Input: part model. Units: mm. Frame: model coordinates. A direction names the side the tool comes from. Coordinates: 2 decimals unless noted, no trailing zeros. Order: outer loops, then holes, each group sorted by start corner. A loop starts at its lowest first (then second) coordinate and runs counter-clockwise, first axis right, second up. Notation, with made-up numbers: (88, -22.5) - (101, -22.5) arc R16 cw to (101, -13.5) - close; hole circle Ø2 at (-16, 75.5). An arc over 180 degrees is marked (long way). Use a Markdown table: item, result. Add a question column.
Autodesk Inventor part; units mm, degrees
ref_plane "Work Plane1" through (0, 0, 46) normal (1, 0, 0) x (0, 0, -1)
ref_plane "YZ Plane" through (0, 0, 0) normal (1, 0, 0) x (0, 1, 0)
ref_plane "XZ Plane" through (0, 0, 0) normal (0, 1, 0) x (-1, 0, 0)
sketch "Sketch1" plane through (0, 0, 0) normal (0, 1, 0) x (-1, 0, 0)
  line L0 (-66, 49) -> (66, 49)
  line L1 (69, 46) -> (69, -46)
  line L2 (66, -49) -> (-66, -49)
  line L3 (-69, -46) -> (-69, 46)
  line L4 (-69, 49) -> (69, -49) construction
  line L5 (69, 49) -> (-69, -49) construction
  arc A0 (69, 46) -> (66, 49) centre (66, 46) ccw
  arc A1 (-66, 49) -> (-69, 46) centre (-66, 46) ccw
  arc A2 (-69, -46) -> (-66, -49) centre (-66, -46) ccw
  arc A3 (66, -49) -> (69, -46) centre (66, -46) ccw
  line L6 (65.5, -42.5) -> (65.5, 42.5)
  line L7 (62.5, 45.5) -> (-62.5, 45.5)
  line L8 (-65.5, 42.5) -> (-65.5, -42.5)
  line L9 (-62.5, -45.5) -> (62.5, -45.5)
  arc A4 (65.5, 42.5) -> (62.5, 45.5) centre (62.5, 42.5) ccw
  arc A5 (-62.5, 45.5) -> (-65.5, 42.5) centre (-62.5, 42.5) ccw
  arc A6 (-65.5, -42.5) -> (-62.5, -45.5) centre (-62.5, -42.5) ccw
  arc A7 (62.5, -45.5) -> (65.5, -42.5) centre (62.5, -42.5) ccw
  point P0 (0, 0)
  dimension "d0" = 138
  dimension "d1" = 98
  dimension "d2" = 3
  dimension "d3" = 3.5
  dimension "d4" = 3
extrude "Extrusion1" add sketch "Sketch1" along normal blind 3.5 contours A7 L9 A6 L8 A5 L7 A4 L6
extrude "Extrusion2" add sketch "Sketch1" along normal blind 42
sketch "Sketch2" plane through (0, 3.5, 0) normal (0, 1, 0) x (1, 0, 0)
  circle A0 centre (-14.4905, 21.8769) radius 1.5
  line L0 (-17.4775, 25.0064) -> (63, 25.0064)
  line L1 (-17.4775, -25.0064) -> (-17.4775, 25.0064)
  circle A1 centre (-14.4905, -22.0231) radius 1.5
  line L2 (63, -25.0064) -> (-17.4775, -25.0064)
  circle A2 centre (60.3095, -22.0231) radius 1.5
  line L3 (63, 25.0064) -> (63, -25.0064)
  circle A3 centre (60.3095, 21.8769) radius 1.5
  line L4 (-62.5, -45.5) -> (62.5, -45.5)
  circle A4 centre (-14.4905, -22.0231) radius 4.5
  circle A5 centre (-14.4905, 21.8769) radius 4.5
  circle A6 centre (60.3095, 21.8769) radius 4.5
  circle A7 centre (60.3095, -22.0231) radius 4.5
  arc A8 (-65.5, -42.5) -> (-62.5, -45.5) centre (-62.5, -42.5) ccw
  line L5 (-62.5, -45.5) -> (62.5, -45.5)
  arc A9 (62.5, -45.5) -> (65.5, -42.5) centre (62.5, -42.5) ccw
  line L6 (65.5, -42.5) -> (65.5, 42.5)
  arc A10 (65.5, 42.5) -> (62.5, 45.5) centre (62.5, 42.5) ccw
  line L7 (62.5, 45.5) -> (-62.5, 45.5)
  arc A11 (-62.5, 45.5) -> (-65.5, 42.5) centre (-62.5, 42.5) ccw
  line L8 (-65.5, 42.5) -> (-65.5, -42.5)
  line L9 (-65.5, -42.5) -> (-65.5, 42.5)
  line L10 (-65.5, 0) -> (-27.8028, 0)
  point P0 (0, 0)
  point P1 (22.7612, -25.0064)
  point P2 (-17.4775, 0)
  dimension "d9" = 3
  dimension "d10" = 80.4775
  dimension "d11" = 50.0127
  dimension "d14" = 2.6905
  dimension "d15" = 46.8833
  dimension "d16" = 2.6905
  dimension "d17" = 2.9833
  dimension "d18" = 77.4905
  dimension "d19" = 46.8833
  dimension "d20" = 77.4905
  dimension "d21" = 2.9833
  dimension "d23" = 9
  dimension "d24" = 9
  dimension "d25" = 9
  dimension "d26" = 9
  dimension "d59" = 2.5
extrude "Extrusion3" add sketch "Sketch2" along normal blind 15 contours L1 A5 L0 | L0 A5 L1 | A6 L3 L0 | L0 L3 A6 | A4 L2 L1 | L1 L2 A4 | A7 L2 L3 | L3 L2 A7
sketch "Sketch4" plane through (0, 3.5, 0) normal (0, 1, 0) x (1, 0, 0)
  circle A0 centre (-43.1118, 27.6225) radius 1.5
  circle A1 centre (-43.1118, -27.6225) radius 1.5
  circle A2 centre (-25.6112, -27.6225) radius 1.4605
  circle A3 centre (-60.6124, 27.6225) radius 1.4605
  line L0 (-30.3737, -42.9768) -> (-36.7237, -42.9768)
  line L1 (-55.8383, 42.9768) -> (-49.4883, 42.9768)
  line L2 (-23.2236, -13.1064) -> (-23.2236, 13.1572)
  line L3 (-63, 13.1572) -> (-63, -13.1064)
  line L4 (-65.5, 42.5) -> (-65.5, -42.5)
  line L5 (-65.5, 0) -> (-9.8345, 0)
  line L6 (-43.1118, -27.6225) -> (-43.1118, 27.6225)
  circle A4 centre (-60.6124, -27.6225) radius 1.4605
  circle A5 centre (-25.6112, 27.6225) radius 1.4605
  circle A6 centre (-60.6124, 32.6225) radius 3.5
  circle A7 centre (-60.6124, -32.6225) radius 3.5
  circle A8 centre (-25.6112, 32.6225) radius 3.5
  circle A9 centre (-25.6112, -32.6225) radius 3.5
  circle A10 centre (-43.1118, -27.6225) radius 4.5
  circle A11 centre (-43.1118, 27.6225) radius 4.5
  point P0 (0, 0)
  point P1 (-43.1997, -2.4081)
  point P2 (-43.1118, 0)
  dimension "d35" = 2.921
  dimension "d36" = 3
  dimension "d37" = 39.7764
  dimension "d38" = 85.9536
  dimension "d41" = 56.134
  dimension "d42" = 29.8704
  dimension "d43" = 2.3876
  dimension "d44" = 15.3543
  dimension "d45" = 7.1501
  dimension "d46" = 13.5001
  dimension "d47" = 19.8882
  dimension "d48" = 70.5993
  dimension "d49" = 19.8882
  dimension "d50" = 15.3543
  dimension "d51" = 19.9761
  dimension "d52" = 40.5687
  dimension "d53" = 26.2647
  dimension "d54" = 32.6147
  dimension "d55" = 37.3888
  dimension "d56" = 70.5993
  dimension "d57" = 56.134
  dimension "d58" = 29.8704
  dimension "d60" = 2.5
  dimension "d61" = 7
  dimension "d62" = 5
  dimension "d63" = 9
  dimension "d64" = 9
extrude "Extrusion5" add sketch "Sketch4" along normal blind 15 contours A11 | A10 | A6 | A7 | A8 | A9
sketch "Sketch5" plane through (0, 3.5, 0) normal (0, 1, 0) x (1, 0, 0)
  circle A0 centre (0, 0) radius 9.75
  circle A1 centre (38.1, 0) radius 15.5
  circle A2 centre (-38.1, 0) radius 15.5
  dimension "d67" = 19.5
  dimension "d68" = 31
  dimension "d69" = 31
  dimension "d70" = 38.1
  dimension "d71" = 38.1
extrude "Extrusion6" cut sketch "Sketch5" against normal through all
ref_plane "Work Plane1" through (0, 0, 46) normal (1, 0, 0) x (0, 0, -1)
sketch "Sketch8" plane through (62.5, 3.5, 45.5) normal (0, 0, -1) x (-1, 0, 0)
  line L0 (-6.5, -3.5) -> (-6.5, 38.5)
  line L1 (6.6905, 15) -> (-2.3095, 15)
  circle A0 centre (16.5, 27) radius 9.75
  line L2 (0, 0) -> (0, 38.5)
  point P0 (62.5, -3.5)
  dimension "d83" = 19.5
  dimension "d84" = 12
  dimension "d87" = 16.5
extrude "Extrusion8" cut sketch "Sketch8" against normal through all
sketch "Sketch9" plane through (0, 3.5, 0) normal (0, 1, 0) x (1, 0, 0)
  circle A0 centre (0, -41) radius 1.5
  circle A1 centre (0, -41) radius 4.5
  line L0 (62.5, -45.5) -> (-62.5, -45.5)
  line L1 (-4.5, -41) -> (-4.5, -45.5)
  line L2 (4.5, -41) -> (4.5, -45.5)
  line L3 (-65.5, -42.5) -> (-65.5, 42.5)
  line L4 (-65.5, 0) -> (0, 0)
  circle A2 centre (0, 41) radius 1.5
  circle A3 centre (0, 41) radius 4.5
  line L5 (-4.5, 41) -> (-4.5, 45.5)
  line L6 (4.5, 41) -> (4.5, 45.5)
  line L7 (-62.5, 45.5) -> (62.5, 45.5)
  dimension "d88" = 3
  dimension "d89" = 9
  dimension "d90" = 4.5
extrude "Extrusion9" add sketch "Sketch9" along normal up to surface (38.5 mm away)
equation "\"d0\" = BoxL"
equation "\"d1\" = BoxW"
equation "\"d2\" = BoxCorner"
equation "\"d3\" = BoxWall"
equation "\"d4\" = BoxCorner"
equation "\"d7\" = BoxH"
equation "\"BoxW\" = 98"
equation "\"BoxL\" = 138"
equation "\"BoxCorner\" = 3"
equation "\"BoxWall\" = 3.5"
equation "\"BoxH\" = 42"
equation "\"PinH\" = 15"
properties part number "Box"
1) Contact query for flat-ended pins moving along their axis: P1, Ø3.5, axis at x = 60, z = 22.5, coming from the +Y side; P2, Ø8, axis at x = 43, y = 28.5, coming from the +Z side; P3, Ø2.5, axis at x = 60.31, z = -21.88, coming from the +Y side. Output: stop coordinate, or through.
2) Pull-direction query (Z, two-part tool) for faces 1 (the cylindrical face through (68.14, 20.71, 48.1)), 2 (the flat face through (69, 21, -1)), 3 (the cylindrical face through (-13.06, 10.9, -21.43)); classes: pulls with the +Z half, pulls with the -Z half, needs draft (parallel to the pull), parting line crosses it, or undercut.
3) Material intervals for L1, parallel to X at y = 1.45, z = 0; L2, parallel to Z at x = 0, y = 17; L3, parallel to X at y = 17, z = 41, sorted ascending.
4) Cut plane C-C (y = 14). State how many separate pieces and enclosed holes the cut face has, and give its area (3 significant figures).
5) Cut plane A-A (x = 0). Return the cut outline in (y, z).
6) Cut plane B-B (x = 46). Return the cut outline in (y, z), and give its area (3 significant figures).
7) Reachability of faces 4 (the flat face through (-43, 3.5, -28)), 5 (the cylindrical face through (52.884, 1.774, -4.656)) from +Z, -Z, +X, -X, +Y, -Y: full face, straight path, thin tool, end or side. Return the list, or none.
Computed:
| question | item | result |
|---|---|---|
| 1 | P1 | stops at y = 18.5 |
| 1 | P2 | stops at z = -45.5 |
| 1 | P3 | stops at y = 3.5 |
| 2 | face 1 | pulls with the +Z half |
| 2 | face 2 | needs draft |
| 2 | face 3 | undercut |
| 3 | L1 | x = -69 to -53.6, -22.6 to -9.75, 9.75 to 22.6, 53.6 to 69 |
| 3 | L2 | z = -49 to -42.5, -39.5 to -36.5, 36.5 to 39.5, 42.5 to 49 |
| 3 | L3 | x = -69 to -65.5, -4.5 to -1.5, 1.5 to 4.5, 65.5 to 69 |
| 4 | separate pieces | 11 |
| 4 | enclosed holes | 9 |
| 4 | area | 2,230 mm2 |
| 5 | outline | (0, -49) - (42, -49) - (42, -42.5) - (3.5, -42.5) - (3.5, -39.5) - (42, -39.5) - (42, -36.5) - (3.5, -36.5) - (3.5, -9.75) - (0, -9.75) - close; (0, 9.75) - (3.5, 9.75) - (3.5, 36.5) - (42, 36.5) - (42, 39.5) - (3.5, 39.5) - (3.5, 42.5) - (42, 42.5) - (42, 49) - (0, 49) - close |
| 6 | outline | (0, -49) - (42, -49) - (42, -45.5) - (3.5, -45.5) - (3.5, -13.34) - (0, -13.34) - close; (0, 13.34) - (3.5, 13.34) - (3.5, 45.5) - (20.75, 45.5) - (20.75, 49) - (0, 49) - close; (40.25, 45.5) - (42, 45.5) - (42, 49) - (40.25, 49) - close |
| 6 | area | 451 mm2 |
| 7 | face 4 | +Y |
| 7 | face 5 | +Y, -Y |
